from build123d import *

# Parameters (mm, degrees)
SKETCH_1_W          = 60
SKETCH_1_H          = 120
SKETCH_1_R          = 1.6
SKETCH_1_R_2        = 2.15
EXTRUDE_3_DEPTH     = 6
SKETCH_9_R          = 1.6
CUT_EXTRUDE_1_DEPTH = 6
FILLET_1_R          = 10
SKETCH_11_R         = 2.15
CUT_EXTRUDE_2_DEPTH = 6
FILLET_2_R          = 20
SKETCH_12_R         = 1.6
CUT_EXTRUDE_3_DEPTH = 10
SKETCH_13_R         = 1.6
CUT_EXTRUDE_4_DEPTH = 10
EXTRUDE_START       = -6
SKETCH_14_R         = 1.6
EXTRUDE_5_DEPTH     = 6


with BuildPart() as part:
    # 草图1 → 凸台-拉伸3 (new body)
    with BuildSketch(Plane.XY):
        Rectangle(SKETCH_1_W, SKETCH_1_H)
        with Locations((0, 50.5)):
            Circle(SKETCH_1_R, mode=Mode.SUBTRACT)
        with Locations((20, -50)):
            Circle(SKETCH_1_R_2, mode=Mode.SUBTRACT)
        with Locations((-20, -50)):
            Circle(SKETCH_1_R_2, mode=Mode.SUBTRACT)
        with Locations((13.423393759, 42.75)):
            Circle(SKETCH_1_R, mode=Mode.SUBTRACT)
        with Locations((13.423393759, 27.25)):
            Circle(SKETCH_1_R, mode=Mode.SUBTRACT)
        with Locations((0, 19.5)):
            Circle(SKETCH_1_R, mode=Mode.SUBTRACT)
        with Locations((-13.423393759, 27.25)):
            Circle(SKETCH_1_R, mode=Mode.SUBTRACT)
        with Locations((-13.423393759, 42.75)):
            Circle(SKETCH_1_R, mode=Mode.SUBTRACT)
        with BuildLine():
            Line((6, 42), (6, 28))
            ThreePointArc((6, 28), (0, 22), (-6, 28))
            Line((-6, 28), (-6, 42))
            ThreePointArc((-6, 42), (0, 48), (6, 42))
        make_face(mode=Mode.SUBTRACT)
    extrude(amount=EXTRUDE_3_DEPTH)

    # 草图9 → 切除-拉伸1 (cut)
    with BuildSketch(Plane.XY.offset(6)):
        with Locations((20.1, -22)):
            Circle(SKETCH_9_R)
        with Locations((20.1, -2)):
            Circle(SKETCH_9_R)
        with Locations((20.1, -12)):
            Circle(SKETCH_9_R)
        with Locations((-20.1, -2)):
            Circle(SKETCH_9_R)
        with Locations((-20.1, -12)):
            Circle(SKETCH_9_R)
        with Locations((-20.1, -22)):
            Circle(SKETCH_9_R)
    extrude(amount=-CUT_EXTRUDE_1_DEPTH, mode=Mode.SUBTRACT)

    # 圆角1
    fillet_1_edges = [part.edges().sort_by_distance(p)[0] for p in [
        (30, -60, 3),
        (-30, -60, 3),
        (-30, 60, 3),
        (30, 60, 3),
    ]]
    fillet(fillet_1_edges, radius=FILLET_1_R)

    # 草图11 → 切除-拉伸2 (cut)
    with BuildSketch(Plane.XY.offset(6)):
        with BuildLine():
            Line((30, -32), (-30, -32))
            Line((-30, -32), (-30, -50))
            ThreePointArc((-30, -50), (-27.071067812, -57.071067812), (-20, -60))
            Line((-20, -60), (20, -60))
            ThreePointArc((20, -60), (27.071067812, -57.071067812), (30, -50))
            Line((30, -50), (30, -32))
        make_face()
        with Locations((-20, -50)):
            Circle(SKETCH_11_R, mode=Mode.SUBTRACT)
        with Locations((20, -50)):
            Circle(SKETCH_11_R, mode=Mode.SUBTRACT)
    extrude(amount=-CUT_EXTRUDE_2_DEPTH, mode=Mode.SUBTRACT)

    # 圆角2
    fillet_2_edges = [part.edges().sort_by_distance(p)[0] for p in [
        (-30, -32, 3),
        (30, -32, 3),
    ]]
    fillet(fillet_2_edges, radius=FILLET_2_R)

    # 草图12 → 切除-拉伸3 (cut)
    with BuildSketch(Plane(origin=(0, 0, 0), x_dir=(-1, 0, 0), z_dir=(0, 0, -1))):
        with Locations((-20, 50)):
            Circle(SKETCH_12_R)
        with Locations((20, 50)):
            Circle(SKETCH_12_R)
        with Locations((25, 10)):
            Circle(SKETCH_12_R)
        with Locations((-25, 10)):
            Circle(SKETCH_12_R)
    extrude(amount=-CUT_EXTRUDE_3_DEPTH, mode=Mode.SUBTRACT)

    # 草图13 → 切除-拉伸4 (cut)
    with BuildSketch(Plane.XY.offset(6)):
        with Locations((-15.5, 35)):
            Circle(SKETCH_13_R)
        with Locations((-7.75, 48.423393759)):
            Circle(SKETCH_13_R)
        with Locations((7.75, 48.423393759)):
            Circle(SKETCH_13_R)
        with Locations((15.5, 35)):
            Circle(SKETCH_13_R)
        with Locations((7.75, 21.576606241)):
            Circle(SKETCH_13_R)
        with Locations((-7.75, 21.576606241)):
            Circle(SKETCH_13_R)
    extrude(amount=-CUT_EXTRUDE_4_DEPTH, mode=Mode.SUBTRACT)

    # 草图14 → 凸台-拉伸5 (add)
    with BuildSketch(Plane.XY.offset(6).offset(EXTRUDE_START)):
        with Locations((0, 50.5)):
            Circle(SKETCH_14_R)
        with Locations((13.423393759, 42.75)):
            Circle(SKETCH_14_R)
        with Locations((13.423393759, 27.25)):
            Circle(SKETCH_14_R)
        with Locations((0, 19.5)):
            Circle(SKETCH_14_R)
        with Locations((-13.423393759, 27.25)):
            Circle(SKETCH_14_R)
        with Locations((-13.423393759, 42.75)):
            Circle(SKETCH_14_R)
    extrude(amount=EXTRUDE_5_DEPTH)


solid = part.part
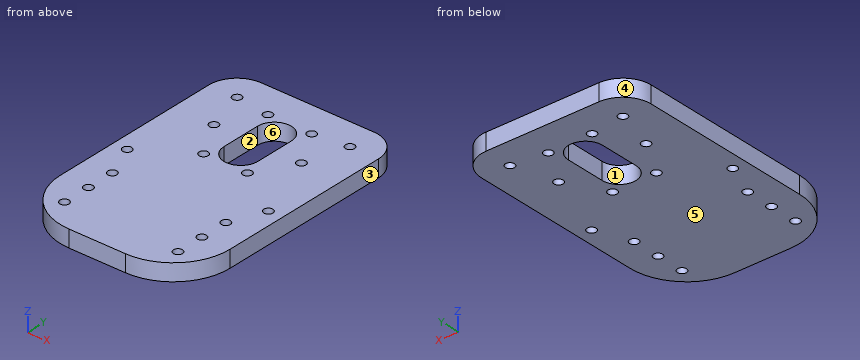
Geometry check sheet. Reference: the model listing, model coordinates, mm. Face numbers are marked on the shaded views. A direction names the side the tool comes from. Round coordinates to 2 decimals unless told otherwise and drop trailing zeros. Write each loop counter-clockwise with the first axis right and the second up, starting at its lowest first coordinate (ties: lowest second). Pieces come first, ordered by that corner, then holes. Notation, with made-up numbers: (17, -16.75) - (27, -16.75) arc R16 ccw to (27, 7.25) - close; hole circle Ø1 at (-3, -14.5). An arc over 180 degrees is marked (long way). One line per item, written item: value.
1. Scan lines: L1, parallel to Y at x = 7.75, z = 3.8; L2, parallel to Y at x = 6.5, z = 5.05; L3, parallel to Y at x = -20, z = 4.45. Record each from-to range of solid material in increasing order.
The answers:
L1: y = -32 to 19.98, 23.18 to 46.82, 50.02 to 60
L2: y = -32 to 20.58, 22.58 to 47.42, 49.42 to 60
L3: y = -29.32 to -23.6, -20.4 to -13.6, -10.4 to -3.6, -0.4 to 48.4, 51.6 to 60
2. Set-up check for the marked faces 5 and 6: record each of +Z, -Z, +X, -X, +Y, -Y from which the full face is reachable in a straight line by a thin tool's end or side.
The answers:
face 5: -Z, +X, -X, +Y, -Y
face 6: +Z, -Z
3. Cross-section at A-A on y = 10. Record the boundary of the cut face in (x, z).
The answers:
outline: (-30, 0) - (-26.6, 0) - (-26.6, 6) - (-30, 6) - close; (-23.4, 0) - (23.4, 0) - (23.4, 6) - (-23.4, 6) - close; (26.6, 0) - (30, 0) - (30, 6) - (26.6, 6) - close
4. Cross-section at B-B on x = 7.75. Record the boundary of the cut face in (y, z).
The answers:
outline: (-32, 0) - (19.98, 0) - (19.98, 6) - (-32, 6) - close; (23.18, 0) - (46.82, 0) - (46.82, 6) - (23.18, 6) - close; (50.02, 0) - (60, 0) - (60, 6) - (50.02, 6) - close
5. Depth check by flat-ended pin: pin 1 Ø4 at (x, y) = (-15.5, 35) entering from +Z; pin 2 Ø1 at (x, z) = (17, 1.5) entering from -Y. Enter the tip coordinate at first touch or a pass-through.
The answers:
pin 1: stops at z = 6
pin 2: stops at y = -30.91
6. Cross-section at C-C on y = 35. Record the boundary of the cut face in (x, z).
The answers:
outline: (-30, 0) - (-17.1, 0) - (-17.1, 6) - (-30, 6) - close; (-13.9, 0) - (-6, 0) - (-6, 6) - (-13.9, 6) - close; (6, 0) - (13.9, 0) - (13.9, 6) - (6, 6) - close; (17.1, 0) - (30, 0) - (30, 6) - (17.1, 6) - close
7. Mould release check, pull along Y, two halves, no side actions. Record for the marked faces 1, 2, 3 and 4: released by +Y, released by -Y, zero draft, split by the parting line, or undercut.
The answers:
face 1: undercut
face 2: undercut
face 3: zero draft
face 4: released by +Y
8. Cross-section at D-D on x = 0. Record the boundary of the cut face in (y, z).
The answers:
outline: (-32, 0) - (22, 0) - (22, 6) - (-32, 6) - close; (48, 0) - (60, 0) - (60, 6) - (48, 6) - close
